Study the drawing (mm; zero at the part's minimum x, y, z) and answer. Coordinates: 2 decimals unless noted, no trailing zeros. Order: outer loops, then holes, each group sorted by start corner. A loop starts at its lowest first (then second) coordinate and runs counter-clockwise, first axis right, second up. Notation, with made-up numbers: M -10.75,33.25 L 13.25,33.25 A3 ccw 13.25,37.25 Z; hole C -25.5,12.5 d5. An arc over 180 degrees is marked long. Use a Markdown table: item, result. Add a question column.
1) Find section C-C on z = 1.5. Count the separate pieces of the cut face and the enclosed holes in it.
2) Find the intervals of material crossed by probe 1 along Y at (x, z) = (54.61, 4) (1 decimal); probe 2 along X at (y, z) = (26, 4.25) (1 decimal); probe 3 along X at (y, z) = (27.5, 1.75) (1 decimal), in increasing order. Write a range as [from, to].
3) Find section A-A on y = 54.61. Write down the section's boundary in (x, z) (1 decimal), plus the area to 3 significant figures.
4) Each of these flat-tipped pins is pushed along its axis until it touches: pin 1 Ø3 at (y, z) = (29.5, 1) entering from -X; pin 2 Ø3 at (x, z) = (91, 4) entering from -Y; pin 3 Ø3 at (x, z) = (66.5, 1.5) entering from -Y. Where does it stop, or does it pass through?
5) The mould has two halves that part along Y. Classify the marked faces 1, 2 and 3: released by +Y, released by -Y, zero draft, split by the parting line, or undercut.
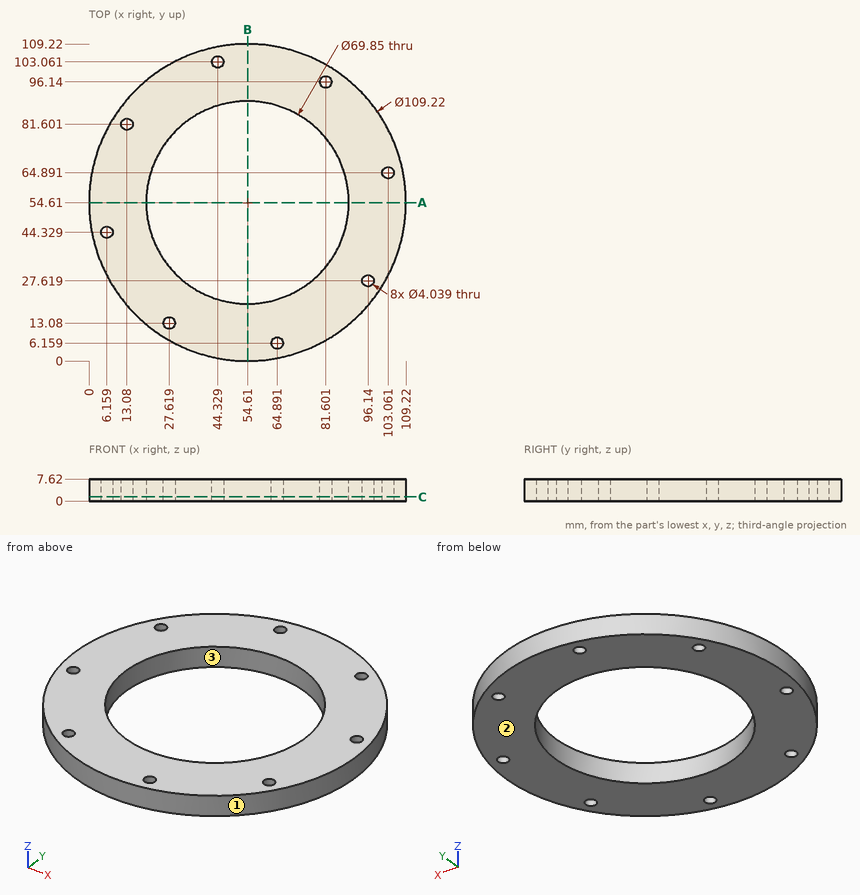
Check result:
| question | item | result |
|---|---|---|
| 1 | separate pieces | 1 |
| 1 | enclosed holes | 9 |
| 2 | probe 1 | y = [0, 19.7], [89.5, 109.2] |
| 2 | probe 2 | x = [8.1, 34.6], [74.6, 94.9], [97.3, 101.1] |
| 2 | probe 3 | x = [7.2, 32.6], [76.6, 94.1], [98.2, 102] |
| 3 | outline | M 0,0 L 19.7,0 L 19.7,7.6 L 0,7.6 Z; M 89.5,0 L 109.2,0 L 109.2,7.6 L 89.5,7.6 Z |
| 3 | area | 300 mm2 |
| 4 | pin 1 | stops at x = 5.37 |
| 4 | pin 2 | stops at y = 12.6 |
| 4 | pin 3 | stops at y = 1 |
| 5 | face 1 | split by the parting line |
| 5 | face 2 | zero draft |
| 5 | face 3 | undercut |
